Read the model definition and answer for the solid it produces. Units are mm, in the model's axes. Face numbers are marked on the shaded views. A direction names the side the tool comes from. Coordinates: 2 decimals unless noted, no trailing zeros. Write each loop counter-clockwise with the first axis right and the second up, starting at its lowest first coordinate (ties: lowest second). Pieces come first, ordered by that corner, then holes. Notation, with made-up numbers: (47, 65) - (85, 65) arc R12 ccw to (85, 84) - close; hole circle Ø3 at (-28.5, 71.25). An arc over 180 degrees is marked (long way). Use a Markdown table: item, result.
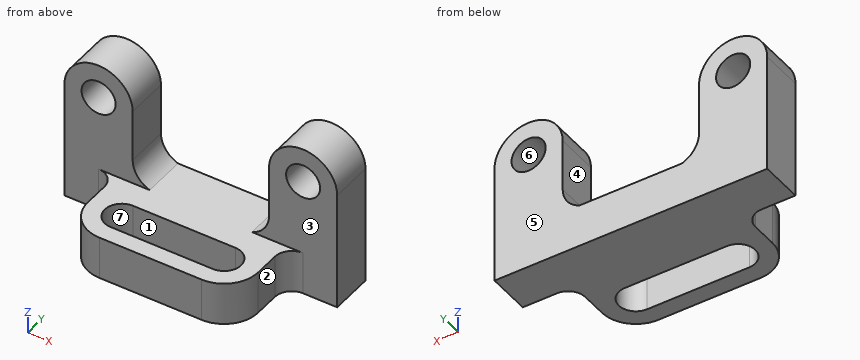
from build123d import *

# Parameters (mm, degrees)
F1_DEPTH = 16.002
F2_R     = 6.35
F3_DEPTH = 16.003
F6_DEPTH = 16.002
F4_W     = 38.1
F4_H     = 12.7
F7_DEPTH = 16.003


# Not quite as in the source:
# - a feature names something its author has since deleted; it is built from what else it names


with BuildPart() as f1:
    # F0 (on Front) → F1 (new body)
    with BuildSketch(Plane.XZ):
        with BuildLine():
            Line((0, 44.45), (0, 0))
            Line((0, 0), (101.6, 0))
            Line((101.6, 0), (101.6, 44.45))
            Line((101.6, 44.45), (76.2, 44.45))
            Line((76.2, 44.45), (76.2, 25.0716141042))
            ThreePointArc((76.2, 25.0716141042), (74.4547062675, 19.535812446), (69.85, 16.002))
            Line((69.85, 16.002), (31.75, 16.002))
            ThreePointArc((31.75, 16.002), (27.1452937325, 19.535812446), (25.4, 25.0716141042))
            Line((25.4, 25.0716141042), (25.4, 44.45))
            Line((25.4, 44.45), (0, 44.45))
        make_face()
        with BuildLine():
            ThreePointArc((25.4, 44.45), (12.7, 57.15), (0, 44.45))
            Line((0, 44.45), (25.4, 44.45))
        make_face()
        with BuildLine():
            Line((76.2, 44.45), (101.6, 44.45))
            ThreePointArc((101.6, 44.45), (88.9, 57.15), (76.2, 44.45))
        make_face()
    extrude(amount=F1_DEPTH)

    # F2 (on face) → F3 (cut, through all)
    with BuildSketch(Plane.XZ.offset(16.002)):
        with Locations((12.7, 44.45)):
            Circle(F2_R)
        with Locations((88.9, 44.45)):
            Circle(F2_R)
    extrude(amount=-F3_DEPTH, mode=Mode.SUBTRACT)

    # F5 (on Top) → F6 (join)
    with BuildSketch(Plane.XY):
        with BuildLine():
            ThreePointArc((19.05, -31.75), (22.7697438789, -40.7302561211), (31.75, -44.45))
            Line((31.75, -44.45), (69.85, -44.45))
            ThreePointArc((69.85, -44.45), (78.8302561211, -40.7302561211), (82.55, -31.75))
            Line((82.55, -31.75), (82.55, -22.352))
            Line((82.55, -22.352), (82.55, -16.002))
            Line((82.55, -16.002), (19.05, -16.002))
            Line((19.05, -16.002), (19.05, -22.352))
            Line((19.05, -22.352), (19.05, -31.75))
        make_face()
        with BuildLine():
            ThreePointArc((12.7, -16.002), (17.1901280605, -17.8618719395), (19.05, -22.352))
            Line((19.05, -22.352), (19.05, -16.002))
            Line((19.05, -16.002), (12.7, -16.002))
        make_face()
        with BuildLine():
            Line((82.55, -16.002), (82.55, -22.352))
            ThreePointArc((82.55, -22.352), (84.4098719395, -17.8618719395), (88.9, -16.002))
            Line((88.9, -16.002), (82.55, -16.002))
        make_face()
    extrude(amount=F6_DEPTH)

    # F4 (on face) → F7 (cut, through all)
    with BuildSketch(Plane.XY.offset(16.002)):
        with Locations((50.8, -31.75)):
            Rectangle(F4_W, F4_H)
        with BuildLine():
            Line((31.75, -38.1), (31.75, -25.4))
            ThreePointArc((31.75, -25.4), (25.4, -31.75), (31.75, -38.1))
        make_face()
        with BuildLine():
            ThreePointArc((69.85, -38.1), (76.2, -31.75), (69.85, -25.4))
            Line((69.85, -25.4), (69.85, -38.1))
        make_face()
    extrude(amount=-F7_DEPTH, mode=Mode.SUBTRACT)


solid = f1.part
(1) A cutting plane is placed at A-A, the plane z = 28. Write down the section's boundary in (x, y), and give its area (3 significant figures).
Report:
| item | result |
|---|---|
| outline | (0, -16) - (25.4, -16) - (25.4, 0) - (0, 0) - close; (76.2, -16) - (101.6, -16) - (101.6, 0) - (76.2, 0) - close |
| area | 813 mm² |
(2) Each of these flat-tipped pins is pushed along its axis until it touches: P1, Ø10, axis at x = 88.9, z = 44.45, coming from the +Y side; P2, Ø3, axis at y = -10.5, z = 49, coming from the +X side; P3, Ø16, axis at x = 19, z = 16.5, coming from the -Y side; P4, Ø3, axis at y = -28.5, z = 9.5, coming from the +X side. Where does it stop, or does it pass through?
Report:
| item | result |
|---|---|
| P1 | passes through |
| P2 | stops at x = 101.23 |
| P3 | stops at y = -43.52 |
| P4 | stops at x = 82.55 |
(3) For the marked faces 1, 2, 3 and 4, determine the directions among +Z, -Z, +X, -X, +Y, -Y from which every point of the face is accessible in a straight line to the end or side of a thin tool.
Report:
| item | result |
|---|---|
| face 1 | +Z, -Z |
| face 2 | +Z, -Z, +X, -Y |
| face 3 | +Z, +X, -Y |
| face 4 | +Z, +Y, -Y |
(4) The mould has two halves that part along Y. Classify the marked faces 5, 6 and 7: pulls with the +Y half, pulls with the -Y half, needs draft (parallel to the pull), parting line crosses it, or undercut.
Report:
| item | result |
|---|---|
| face 5 | pulls with the +Y half |
| face 6 | needs draft |
| face 7 | undercut |
(5) A cutting plane is placed at C-C, the plane x = 29.5. Write down the section's boundary in (y, z), and give its area (3 significant figures).
Report:
| item | result |
|---|---|
| outline | (-44.25, 0) - (-37.69, 0) - (-37.69, 16) - (-44.25, 16) - close; (-25.81, 0) - (0, 0) - (0, 17.18) - (-16, 17.18) - (-16, 16) - (-25.81, 16) - close |
| area | 537 mm² |
(6) Straight lines are drawn through the part: L1, parallel to Y at x = 36, z = 3; L2, parallel to Z at x = 88.9, y = -10; L3, parallel to X at y = -7.5, z = 33. For each, find the intervals that lie inside material, in ascending order.
Report:
| item | result |
|---|---|
| L1 | y = -44.45 to -38.1, -25.4 to 0 |
| L2 | z = 0 to 38.1, 50.8 to 57.15 |
| L3 | x = 0 to 25.4, 76.2 to 101.6 |
(7) A cutting plane is placed at B-B, the plane x = 58.5. Write down the section's boundary in (y, z).
Report:
| item | result |
|---|---|
| outline | (-44.45, 0) - (-38.1, 0) - (-38.1, 16) - (-44.45, 16) - close; (-25.4, 0) - (0, 0) - (0, 16) - (-25.4, 16) - close |
